Geometry check sheet. Reference: the model listing, model coordinates, mm. Face numbers are marked on the shaded views. A direction names the side the tool comes from. Coordinates: 2 decimals unless noted, no trailing zeros. Write each loop counter-clockwise with the first axis right and the second up, starting at its lowest first coordinate (ties: lowest second). Pieces come first, ordered by that corner, then holes.
from build123d import *

# Parameters (mm, degrees)
SKETCH_W        = 80
SKETCH_H        = 80
PAD_DEPTH       = 50
SKETCH007_W     = 13.4
SKETCH007_H     = 13.4
SKETCH007_R     = 3.25
POCKET_DEPTH    = 5
SKETCH004_R     = 2.45
PAD001_DEPTH    = 3
POCKET001_DEPTH = 40
POCKET002_DEPTH = 10.001
SKETCH002_W     = 48.1
SKETCH002_H     = 4
POCKET003_DEPTH = 80.001
SKETCH003_W     = 48.1
SKETCH003_H     = 4
POCKET004_DEPTH = 80.001


with BuildPart() as part:
    # Sketch → Pad (new body)
    with BuildSketch(Plane.XY):
        Rectangle(SKETCH_W, SKETCH_H)
    extrude(amount=PAD_DEPTH)

    # Sketch007 → Pocket (cut)
    with BuildSketch(Plane(origin=(0, 0, 0), x_dir=(1, 0, 0), z_dir=(0, 0, -1))):
        with Locations((-31.95, 31.95)):
            Rectangle(SKETCH007_W, SKETCH007_H)
        with Locations((-31.95, 31.95)):
            Circle(SKETCH007_R, mode=Mode.SUBTRACT)
        with Locations((31.95, 31.95)):
            Rectangle(SKETCH007_W, SKETCH007_H)
        with Locations((31.95, 31.95)):
            Circle(SKETCH007_R, mode=Mode.SUBTRACT)
        with Locations((-31.95, -31.95)):
            Rectangle(SKETCH007_W, SKETCH007_H)
        with Locations((-31.95, -31.95)):
            Circle(SKETCH007_R, mode=Mode.SUBTRACT)
        with Locations((31.95, -31.95)):
            Rectangle(SKETCH007_W, SKETCH007_H)
        with Locations((31.95, -31.95)):
            Circle(SKETCH007_R, mode=Mode.SUBTRACT)
    extrude(amount=-POCKET_DEPTH, mode=Mode.SUBTRACT)

    # Sketch004 → Pad001 (new body)
    with BuildSketch(Plane.XY.offset(50)):
        with Locations((-35.95, -35.95)):
            Circle(SKETCH004_R)
        with Locations((35.95, 35.95)):
            Circle(SKETCH004_R)
        with Locations((35.95, -35.95)):
            Circle(SKETCH004_R)
        with Locations((-35.95, 35.95)):
            Circle(SKETCH004_R)
        with Locations((-27.95, 35.95)):
            Circle(SKETCH004_R)
        with Locations((-27.95, 27.95)):
            Circle(SKETCH004_R)
        with Locations((27.95, 27.95)):
            Circle(SKETCH004_R)
        with Locations((27.95, 35.95)):
            Circle(SKETCH004_R)
        with Locations((-35.95, 27.95)):
            Circle(SKETCH004_R)
        with Locations((35.95, 27.95)):
            Circle(SKETCH004_R)
        with Locations((27.95, -27.95)):
            Circle(SKETCH004_R)
        with Locations((27.95, -35.95)):
            Circle(SKETCH004_R)
        with Locations((35.95, -27.95)):
            Circle(SKETCH004_R)
        with Locations((-27.95, -27.95)):
            Circle(SKETCH004_R)
        with Locations((-27.95, -35.95)):
            Circle(SKETCH004_R)
        with Locations((-35.95, -27.95)):
            Circle(SKETCH004_R)
    extrude(amount=PAD001_DEPTH)

    # Sketch008 → Pocket001 (cut)
    with BuildSketch(Plane.XY.offset(50)):
        Polygon((-24, 40), (-24, 24), (-40, 24), (-40, -24), (-24, -24), (-24, -40), (24, -40), (24, -24), (40, -24), (40, 24), (24, 24), (24, 40), align=None)
    extrude(amount=-POCKET001_DEPTH, mode=Mode.SUBTRACT)

    # Sketch005 → Pocket002 (cut, through all)
    with BuildSketch(Plane.XY.offset(10)):
        Polygon((24, 24), (24, 32), (-24, 32), (-24, 24), (-32, 24), (-32, -24), (-24, -24), (-24, -32), (24, -32), (24, -24), (40, -24), (40, 24), align=None)
    extrude(amount=-POCKET002_DEPTH, mode=Mode.SUBTRACT)

    # Sketch002 → Pocket003 (cut, through all)
    with BuildSketch(Plane.XZ.offset(40)):
        with Locations((0, 2)):
            Rectangle(SKETCH002_W, SKETCH002_H)
    extrude(amount=-POCKET003_DEPTH, mode=Mode.SUBTRACT)

    # Sketch003 → Pocket004 (cut, through all)
    with BuildSketch(Plane(origin=(-40, 0, 0), x_dir=(0, -1, 0), z_dir=(-1, 0, 0))):
        with Locations((0, 2)):
            Rectangle(SKETCH003_W, SKETCH003_H)
    extrude(amount=-POCKET004_DEPTH, mode=Mode.SUBTRACT)


solid = part.part
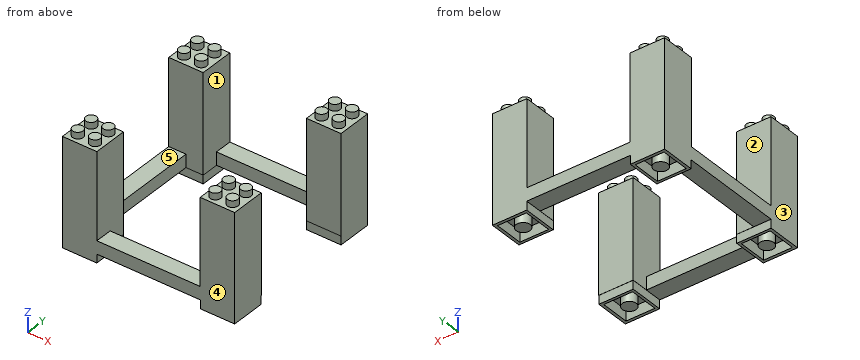
1. Access from +Z, -Z, +X, -X, +Y, -Y to the whole of each face (thin tool, end or side, straight path). Record for the marked faces 4 and 5.
Computed values:
face 4: +Z, -Z, +X, -X, -Y
face 5: +Z, +X, -X
2. Sectioned sample at B-B, the plane x = -20.5. Record the boundary of the cut face in (y, z).
Computed values:
outline: (-40, 4) - (-32, 4) - (-32, 10) - (-40, 10) - close; (32, 4) - (40, 4) - (40, 10) - (32, 10) - close
3. Sectioned sample at C-C, the plane y = 3. Record the boundary of the cut face in (x, z), and give its area (3 significant figures).
Computed values:
outline: (-40, 4) - (-32, 4) - (-32, 10) - (-40, 10) - close
area: 48.0 mm2
4. Sectioned sample at A-A, the plane z = 39.5. Record the boundary of the cut face in (x, y).
Computed values:
outline: (-40, -40) - (-24, -40) - (-24, -24) - (-40, -24) - close; (-40, 24) - (-24, 24) - (-24, 40) - (-40, 40) - close; (24, -40) - (40, -40) - (40, -24) - (24, -24) - close; (24, 24) - (40, 24) - (40, 40) - (24, 40) - close
5. Thickness scan on line 1 along X through (y, z) = (29, 44.5); line 2 along Z through (x, y) = (-35.5, 13.5). Record the ranges inside material, lowest first.
Computed values:
line 1: x = -40 to -24, 24 to 40
line 2: z = 4 to 10
6. Draft check along X on the marked faces 1, 2 and 3. Enter one of: released by +X, released by -X, zero draft, split by the parting line, or undercut.
Computed values:
face 1: undercut
face 2: zero draft
face 3: released by -X
7. Gauge pin test, flat ends, axial feed: pin 1 Ø4 at (x, y) = (-34, 10.5) entering from +Z; pin 2 Ø3 at (y, z) = (-4.5, 7) entering from +X; pin 3 Ø12 at (x, y) = (-32, -13.5) entering from -Z. Record the tip position at first contact, or that the pin passes through.
Computed values:
pin 1: stops at z = 10
pin 2: stops at x = -32
pin 3: stops at z = 4
